```python
from build123d import *

# Parameters (mm, degrees)
F1_DEPTH  = 102
F2_W      = 290
F2_H      = 1
F3_DEPTH  = 57.5
F2_R      = 4
F4_DEPTH  = 1
F5_W      = 3
F5_H      = 1.5
F6_DEPTH  = 1
F7_R      = 5
F8_DEPTH  = 1
F10_DEPTH = 61


with BuildPart() as f1:
    # F0 (on Top) → F1 (new body)
    with BuildSketch(Plane.XY):
        Polygon((-146, 60), (-146, 0), (-137, 0), (-137, 1), (-145, 1), (-145, 2.5), (-137, 2.5), (-137, 3.5), (-145, 3.5), (-145, 61), (-161, 61), (-161, 60), align=None)
    extrude(amount=F1_DEPTH)



with BuildPart() as f1b:
    # F0 (on Top) → F1, piece 2 (new body)
    with BuildSketch(Plane.XY):
        Polygon((137, 1), (137, 0), (146, 0), (146, 60), (161, 60), (161, 61), (145, 61), (145, 3.5), (137, 3.5), (137, 2.5), (145, 2.5), (145, 1), align=None)
    extrude(amount=F1_DEPTH)


with BuildPart() as f1_1:
    add(f1.part)

    add(f1b.part)  # F3 merges F1b
    # F2 (on face) → F3 (join)
    with BuildSketch(Plane(origin=(0, 61, 0), x_dir=(-1, 0, 0), z_dir=(0, 1, 0))):
        with Locations((0, 101.5)):
            Rectangle(F2_W, F2_H)
        with Locations((0, 0.5)):
            Rectangle(F2_W, F2_H)
    extrude(amount=-F3_DEPTH)

    # F2 (on face) → F4 (cut, through all)
    with BuildSketch(Plane(origin=(0, 61, 0), x_dir=(-1, 0, 0), z_dir=(0, 1, 0))):
        with Locations((-152.5, 76.5)):
            Circle(F2_R)
        with Locations((-152.5, 51)):
            Circle(F2_R)
        with Locations((-152.5, 25.5)):
            Circle(F2_R)
        with Locations((152.5, 76.5)):
            Circle(F2_R)
        with Locations((152.5, 51)):
            Circle(F2_R)
        with Locations((152.5, 25.5)):
            Circle(F2_R)
    extrude(amount=-F4_DEPTH, mode=Mode.SUBTRACT)

    # F5 (on face) → F6 (join)
    with BuildSketch(Plane(origin=(0, 0, 0), x_dir=(1, 0, 0), z_dir=(0, 0, -1))):
        with Locations((-143.5, -1.75)):
            Rectangle(F5_W, F5_H)
        with Locations((143.5, -1.75)):
            Rectangle(F5_W, F5_H)
    extrude(amount=-F6_DEPTH)

    # F7 (on face) → F8 (join)
    with BuildSketch(Plane.XZ.offset(-3.5)):
        with BuildLine():
            Line((20, 0), (-20, 0))
            ThreePointArc((-20, 0), (0, -20), (20, 0))
        make_face()
        with Locations((0, -10)):
            Circle(F7_R, mode=Mode.SUBTRACT)
    extrude(amount=-F8_DEPTH)

    # F9 (on Front) → F10 (cut)
    with BuildSketch(Plane.XZ):
        Polygon((48.3850128949, 102.0231251585), (-48.4258194991, 102.1056490811), (-48.4258194991, 100.3182497944), (48.3850128949, 100.3182497944), align=None)
    extrude(amount=-F10_DEPTH, mode=Mode.SUBTRACT)


solid = f1_1.part
```
The listing builds one solid part. Answer for the finished solid, in the listing's coordinates (mm). A direction names the side the tool comes from. Give positions to 0.01 mm unless a question says otherwise; leave off trailing zeros. Loops run counter-clockwise (first coordinate to the right, second up) from the corner with the lowest first, then second, coordinate; pieces in that order, holes last. Notation, with made-up numbers: M 57.25,69.5 L 82.25,69.5 A24 cw 82.25,104.5 Z; hole C 22,70 d4. An arc over 180 degrees is marked long. One line per item, written item: value.
Q1. A cutting plane is placed at A-A on z = 9. Determine the outline of the cut face in (x, y).
Working result:
outline: M -161,60 L -146,60 L -146,0 L -137,0 L -137,1 L -145,1 L -145,2.5 L -137,2.5 L -137,3.5 L -145,3.5 L -145,61 L -161,61 Z; M 137,0 L 146,0 L 146,60 L 161,60 L 161,61 L 145,61 L 145,3.5 L 137,3.5 L 137,2.5 L 145,2.5 L 145,1 L 137,1 Z
Q2. Determine the mould class of faces 1 (the face through (-157, 60, 50)), 2 (the face through (-0.651, 3.993, -5.043)), 3 (the face through (-2, 30, 0)) for opening direction Z: +Z half, -Z half, draft (parallel to the pull), parting line (faces both ways), or undercut.
Working result:
face 1: draft
face 2: undercut
face 3: -Z half
Q3. A cutting plane is placed at C-C on z = 51. Give the number of separate pieces and of enclosed holes in the cut face, then the cut area to 3 significant figures.
Working result:
separate pieces: 4
enclosed holes: 0
area: 168 mm^2
Q4. For faces 4 (the face through (0.6, 3.5, -4.8)), 5 (the face through (141, 2.5, 50)), 6 (the face through (-145, 32, 50)), 7 (the face through (-146, 30, 50)), 8 (the face through (146, 30, 50)), determine the directions among +Z, -Z, +X, -X, +Y, -Y from which every point of the face is accessible in a straight line to the end or side of a thin tool.
Working result:
face 4: +Z, -Z, -Y
face 5: +Z
face 6: +Y
face 7: +Z, -Z, -X, -Y
face 8: +Z, -Z, +X, -Y
Q5. Flat-ended cylindrical pins translate along their axes: P1, Ø1.1, axis at y = 0.5, z = 63, coming from the +X side; P2, Ø12, axis at y = 35.5, z = 55, coming from the -X side; P3, Ø6, axis at x = 15.5, y = 45.5, coming from the -Z side. Find the tip coordinate at first contact, or state that the pin passes through.
Working result:
P1: stops at x = 146
P2: stops at x = -146
P3: stops at z = 0
Q6. A cutting plane is placed at D-D on x = 152.5. Determine the outline of the cut face in (y, z).
Working result:
outline: M 60,0 L 61,0 L 61,21.5 L 60,21.5 Z; M 60,29.5 L 61,29.5 L 61,47 L 60,47 Z; M 60,55 L 61,55 L 61,72.5 L 60,72.5 Z; M 60,80.5 L 61,80.5 L 61,102 L 60,102 Z
Q7. Find the intervals of material crossed by line 1 (Z direction, x = -152.5, y = 60.7); line 2 (X direction, y = 35.5, z = 57); line 3 (Z direction, x = 140, y = 16), in increasing order. Write a range as from..to.
Working result:
line 1: z = 0..21.5, 29.5..47, 55..72.5, 80.5..102
line 2: x = -146..-145, 145..146
line 3: z = 0..1, 101..102
Q8. A cutting plane is placed at B-B on x = 0. Determine the outline of the cut face in (y, z).
Working result:
outline: M 3.5,-20 L 4.5,-20 L 4.5,-15 L 3.5,-15 Z; M 3.5,-5 L 4.5,-5 L 4.5,0 L 61,0 L 61,1 L 3.5,1 Z
